```python
from build123d import *

# Parameters (mm, degrees)
F0_W     = 140
F0_H     = 30
F1_DEPTH = 5
F2_W     = 132
F2_H     = 2.2
F3_DEPTH = 2
F4_W     = 1.375111
F4_H     = 1.664341
F4_W_2   = 1.126474
F4_H_2   = 1.517188
F4_W_3   = 1.309146
F4_H_3   = 2.136242
F5_DEPTH = 1.5


with BuildPart() as f1:
    # F0 (on Top) → F1 (new body)
    with BuildSketch(Plane.XY):
        Rectangle(F0_W, F0_H)
    extrude(amount=F1_DEPTH)

    # F2 (on face) → F3 (cut)
    with BuildSketch(Plane.XY.offset(5)):
        Rectangle(F2_W, F2_H)
    extrude(amount=-F3_DEPTH, mode=Mode.SUBTRACT)

    # F4 (on face) → F5 (join)
    with BuildSketch(Plane.XY.offset(5)):
        Polygon((-62.559685, -11.951999), (-62.559685, -8.897324), (-63.549156, -8.181861), (-62.828619, -7.603401), (-62.828619, -5.583865), (-63.868832, -4.614691), (-67.014842, -4.614691), (-67.014842, -10.937157), (-66, -11.951999), align=None)
        with Locations((-64.7898, -9.729494)):
            Rectangle(F4_W, F4_H, mode=Mode.SUBTRACT)
        with Locations((-64.914119, -6.768693)):
            Rectangle(F4_W_2, F4_H_2, mode=Mode.SUBTRACT)
        Polygon((-57.140429, -4.614691), (-58.738805, -4.614691), (-59.510085, -6.887937), (-60.220474, -4.614691), (-61.808702, -4.614691), (-60.271217, -9.145961), (-61.220094, -11.951999), (-59.616643, -11.951999), align=None)
        Polygon((-54.197387, -11.951999), (-52.654827, -11.951999), (-52.654827, -9.541749), (-51.345681, -9.541749), (-51.345681, -11.951999), (-49.808195, -11.951999), (-49.808195, -4.614691), (-53.015096, -4.614691), (-54.197387, -5.776685), align=None)
        with Locations((-52.000254, -7.07822)):
            Rectangle(F4_W_3, F4_H_3, mode=Mode.SUBTRACT)
        Polygon((-43.541545, -4.614691), (-45.317519, -4.614691), (-46.332361, -8.268122), (-47.347203, -4.614691), (-49.123176, -4.614691), (-49.123176, -11.951999), (-47.702398, -11.951999), (-47.702398, -7.38521), (-46.5607, -11.951999), (-46.104021, -11.951999), (-44.962324, -7.38521), (-44.962324, -11.951999), (-43.541545, -11.951999), align=None)
        Polygon((-37.203856, -4.614691), (-38.97983, -4.614691), (-39.994672, -8.268122), (-41.009514, -4.614691), (-42.785488, -4.614691), (-42.785488, -11.951999), (-41.364709, -11.951999), (-41.364709, -7.38521), (-40.223012, -11.951999), (-39.766333, -11.951999), (-38.624635, -7.38521), (-38.624635, -11.951999), (-37.203856, -11.951999), align=None)
        Polygon((-36.447799, -11.951999), (-34.905239, -11.951999), (-34.905239, -9.541749), (-33.596093, -9.541749), (-33.596093, -11.951999), (-32.058607, -11.951999), (-32.058607, -4.614691), (-35.265508, -4.614691), (-36.447799, -5.776685), align=None)
        with Locations((-34.250666, -7.07822)):
            Rectangle(F4_W_3, F4_H_3, mode=Mode.SUBTRACT)
        Polygon((-28.466066, -4.614691), (-28.466066, -8.826285), (-29.957884, -4.614691), (-31.480147, -4.614691), (-31.480147, -11.951999), (-30.039071, -11.951999), (-30.039071, -7.740404), (-28.537105, -11.951999), (-27.014842, -11.951999), (-27.014842, -4.614691), align=None)
    extrude(amount=F5_DEPTH)


solid = f1.part
```
The listing builds one solid part. Answer for the finished solid, in the listing's coordinates (mm). A direction names the side the tool comes from. Coordinates: 2 decimals unless noted, no trailing zeros. Loops run counter-clockwise (first coordinate to the right, second up) from the corner with the lowest first, then second, coordinate; pieces in that order, holes last. Notation, with made-up numbers: M 38,22.5 L 75,22.5 A30 ccw 75,55.5 Z; hole C 36,-28 d8. An arc over 180 degrees is marked long. Answer as a JSON object with one key per item and string values. Group by question number.
Item 1: Section A-A (x = 22) is taken. Write down the section's boundary in (y, z), and give its area (3 significant figures).
Item 2: Each of these flat-tipped pins is pushed along its axis until it touches: P1, Ø1.6, axis at x = -42.5, z = 6, coming from the +Y side; P2, Ø0.7, axis at x = -27.5, y = 0, coming from the +Z side; P3, Ø0.7, axis at x = -34, z = 5.5, coming from the -Y side. Where does it stop, or does it pass through?
Item 3: Determine the mould class of faces 3 (the face through (-1, 0, 3)), 4 (the face through (-70, 0, 2)), 5 (the face through (-1, 15, 2)), 6 (the face through (-1, -15, 2)) for opening direction Y: +Y half, -Y half, draft (parallel to the pull), parting line (faces both ways), or undercut.
Item 4: Consider L1, parallel to Y at x = 11.5, z = 4; L2, parallel to Z at x = -17.5, y = -11.25; L3, parallel to Y at x = -27.5, z = 5.5. Determine where each line is inside the solid, lowest interval first.
Item 5: Section B-B (y = 5) is taken. Write down the section's boundary in (x, z).
Item 6: Which of the six approach directions +Z, -Z, +X, -X, +Y, -Y give full straight-line access (tool end or side, diameter ignored) to faces 1 (the face through (-1, 0, 0)), 2 (the face through (-58.396, -8.335, 5.74))?
Solved:
{
 "1": {"outline": "M -15,0 L 15,0 L 15,5 L 1.1,5 L 1.1,3 L -1.1,3 L -1.1,5 L -15,5 Z", "area": "146 mm2"},
 "2": {"P1": "stops at y = -4.61", "P2": "stops at z = 3", "P3": "stops at y = -9.54"},
 "3": {"face 3": "undercut", "face 4": "draft", "face 5": "+Y half", "face 6": "-Y half"},
 "4": {"L1": "y = -15 to -1.1, 1.1 to 15", "L2": "z = 0 to 5", "L3": "y = -11.95 to -4.61"},
 "5": {"outline": "M -70,0 L 70,0 L 70,5 L -70,5 Z"},
 "6": {"face 1": "-Z, +X, -X, +Y, -Y", "face 2": "+Z, -Y"}
}
